The model under review builds one solid part; all positions refer to its coordinate system, in mm. A direction names the side the tool comes from. Coordinates: 2 decimals unless noted, no trailing zeros. Order: outer loops, then holes, each group sorted by start corner. A loop starts at its lowest first (then second) coordinate and runs counter-clockwise, first axis right, second up.
Autodesk Inventor part; units mm, degrees
ref_plane "YZ Plane" through (0, 0, 0) normal (1, 0, 0) x (0, 1, 0)
ref_plane "XZ Plane" through (0, 0, 0) normal (0, 1, 0) x (-1, 0, 0)
ref_plane "XY Plane" through (0, 0, 0) normal (0, 0, 1) x (1, 0, 0)
sketch "Sketch1" plane through (0, 0, 0) normal (0, 1, 0) x (-1, 0, 0)
  line L0 (-45.818, 12.7) -> (-187.1472, 12.7)
  arc A0 (-187.1472, 12.7) -> (-190.3222, 9.525) centre (-187.1472, 9.525) ccw
  line L1 (-190.3222, 9.525) -> (-190.3222, -73.025)
  arc A1 (-190.3222, -73.025) -> (-187.1472, -76.2) centre (-187.1472, -73.025) ccw
  line L2 (-187.1472, -76.2) -> (-177.6222, -76.2)
  line L3 (-177.6222, -76.2) -> (-114.1222, -12.7)
  line L4 (-114.1222, -12.7) -> (-45.818, -12.7)
  arc A2 (-31.6867, -16.9939) -> (-45.818, -12.7) centre (-45.818, -38.1) ccw
  line L5 (-31.6867, -16.9939) -> (-17.6641, -26.3826)
  arc A3 (-17.6641, -26.3826) -> (-17.6641, 26.3826) centre (0, 0) ccw
  line L6 (-17.6641, 26.3826) -> (-31.6867, 16.9939)
  arc A4 (-45.818, 12.7) -> (-31.6867, 16.9939) centre (-45.818, 38.1) ccw
  line L7 (-174.4472, -12.7) -> (-134.4873, -12.7)
  arc A5 (-132.2423, -18.1201) -> (-134.4873, -12.7) centre (-134.4873, -15.875) ccw
  line L8 (-132.2423, -18.1201) -> (-172.2021, -58.0799)
  arc A6 (-177.6222, -55.8349) -> (-172.2021, -58.0799) centre (-174.4472, -55.8349) ccw
  line L9 (-177.6222, -55.8349) -> (-177.6222, -15.875)
  arc A7 (-174.4472, -12.7) -> (-177.6222, -15.875) centre (-174.4472, -15.875) ccw
  circle A8 centre (-183.9722, 7.62) radius 2.5527
  circle A9 centre (-183.9722, -68.58) radius 2.5527
  circle A10 centre (-183.9722, -55.88) radius 2.5527
  circle A11 centre (-183.9722, -43.18) radius 2.5527
  circle A12 centre (-183.9722, -30.48) radius 2.5527
  circle A13 centre (-183.9722, -17.78) radius 2.5527
  circle A14 centre (-183.9722, -5.08) radius 2.5527
  circle A15 centre (0, 0) radius 12.827
  circle A16 centre (0, -23.8252) radius 2.5527
  circle A17 centre (-20.6332, -11.9126) radius 2.5527
  circle A18 centre (-20.6332, 11.9126) radius 2.5527
  circle A19 centre (0, 23.8252) radius 2.5527
  circle A20 centre (20.6332, 11.9126) radius 2.5527
  circle A21 centre (20.6332, -11.9126) radius 2.5527
  circle A22 centre (-37.9222, 0) radius 2.5527
  circle A23 centre (-50.6222, 0) radius 2.5527
  circle A24 centre (-63.3222, 0) radius 2.5527
  circle A25 centre (-76.0222, 0) radius 2.5527
  circle A26 centre (-88.7222, 0) radius 2.5527
  circle A27 centre (-101.4222, 0) radius 2.5527
  circle A28 centre (-114.1222, 0) radius 2.5527
  circle A29 centre (-126.8222, 0) radius 2.5527
  circle A30 centre (-139.5222, 0) radius 2.5527
  circle A31 centre (-152.2222, 0) radius 2.5527
  circle A32 centre (-164.9222, 0) radius 2.5527
  circle A33 centre (0, 0) radius 15.9131
  arc A34 (-16.251, -24.272) -> (-16.251, 24.272) centre (0, 0) ccw
  line L10 (-16.251, 24.272) -> (-30.2736, 14.8833)
  line L11 (-30.2736, -14.8833) -> (-16.251, -24.272)
  arc A35 (-45.818, 12.7) -> (-30.2736, 14.8833) centre (-48.2316, 86.3103) ccw
  arc A36 (-30.2736, -14.8833) -> (-45.818, -12.7) centre (-48.2316, -86.3103) ccw
  point P0 (-31.6867, -16.9939)
  point P1 (-17.6641, 26.3826)
  point P2 (-114.1222, -12.7)
  point P3 (-132.2423, -18.1201)
  point P4 (-43.2812, -12.827)
  point P5 (-16.251, 24.272)
  point P6 (-43.2812, 12.827)
  dimension "d1" = 31.8262
  dimension "d2" = 2.54
  dimension "d3" = 2.54
  dimension "d4" = 2.54
extrude "Plate1" add sketch "Sketch1" along normal blind 4.7625 contours A4 A35 L10 A34 L11 A36 A2 L4 L3 L2 A1 L1 A0 L0
equation "\"d0\" = Thickness"
equation "\"BendRadius\" = Thickness"
equation "\"BendReliefWidth\" = Thickness"
equation "\"BendReliefDepth\" = 0.5 * Thickness"
equation "\"CornerReliefSize\" = 4 * Thickness"
equation "\"MinimumRemnant\" = 2 * Thickness"
equation "\"TransitionRadius\" = BendRadius"
equation "\"JacobiRadiusSize\" = BendRadius"
equation "\"GapSize\" = Thickness"
properties part number "climber-arm-brace" material "Aluminum 6061"
(1) Consider section C-C (x = 38). Give the boundary of the cut face in (y, z), then the cut area to 3 significant figures.
(2) Insertion check: pin 1 Ø6 at (x, z) = (63.32, 0) entering from -Y; pin 2 Ø4 at (x, z) = (183.97, -55.88) entering from -Y; pin 3 Ø2 at (x, y) = (166, 1.5) entering from -Z; pin 4 Ø1.4 at (x, y) = (66.5, 2.5) entering from -Z. Each pin has a flat end and moves straight along its axis. Give the tip position at first contact, or say it passes through.
(3) Consider section B-B (z = -43.18). Give the boundary of the cut face in (x, y), then the cut area to 3 significant figures.
(4) Tool access review of faces 4 (the face through (190.322, 2, -31)), 5 (the face through (155, 2, -12.7)): name each direction out of +Z, -Z, +X, -X, +Y, -Y from which nothing blocks a thin tool from reaching the whole face with its end or side.
(5) Consider section D-D (z = 0). Give the number of separate pieces and of enclosed holes in the cut face, then the cut area to 3 significant figures.
(6) Wall thickness on line 1 (Z direction, x = 63.5, y = 3.55); line 2 (Z direction, x = -19, y = 3.25); line 3 (Z direction, x = 93, y = 3.2): over which ranges is each line inside the solid? List them lowest first.
(7) The part is to be moulded in two halves that separate along Z. For faces 1 (the face through (-20.08, 2.35, -9.42)), 2 (the face through (23.164, 2.348, 19.643)), 3 (the face through (80, 2, -12.7)), say which applies: +Z half, -Z half, draft (parallel to the pull), parting line (faces both ways), or undercut.
(8) Consider section A-A (x = 0). Give the boundary of the cut face in (y, z).
Findings:
1. outline: (0, -13.37) - (4.76, -13.37) - (4.76, -2.55) - (0, -2.55) - close; (0, 2.55) - (4.76, 2.55) - (4.76, 13.37) - (0, 13.37) - close
1. area: 103 mm2
2. pin 1: stops at y = 0
2. pin 2: passes through
2. pin 3: stops at z = -65.58
2. pin 4: stops at z = -12.7
3. outline: (144.6, 0) - (157.3, 0) - (157.3, 4.76) - (144.6, 4.76) - close; (177.62, 0) - (181.42, 0) - (181.42, 4.76) - (177.62, 4.76) - close; (186.52, 0) - (190.32, 0) - (190.32, 4.76) - (186.52, 4.76) - close
3. area: 96.7 mm2
4. face 4: +Z, -Z, +X, +Y, -Y
4. face 5: +Y, -Y
5. separate pieces: 13
5. enclosed holes: 0
5. area: 626 mm2
6. line 1: z = -12.7 to -2.55, 2.55 to 12.7
6. line 2: z = -22.19 to -13.87, -9.95 to 9.95, 13.87 to 22.19
6. line 3: z = -12.7 to 12.7
7. face 1: undercut
7. face 2: +Z half
7. face 3: -Z half
8. outline: (0, -29.21) - (4.76, -29.21) - (4.76, -26.38) - (0, -26.38) - close; (0, -21.27) - (4.76, -21.27) - (4.76, -15.91) - (0, -15.91) - close; (0, 15.91) - (4.76, 15.91) - (4.76, 21.27) - (0, 21.27) - close; (0, 26.38) - (4.76, 26.38) - (4.76, 29.21) - (0, 29.21) - close
